Part model, mm, in its own coordinate system. A direction names the side the tool comes from. Give positions to 0.01 mm unless a question says otherwise; leave off trailing zeros. Order: outer loops, then holes, each group sorted by start corner. A loop starts at its lowest first (then second) coordinate and runs counter-clockwise, first axis right, second up. Notation, with made-up numbers: M -19,-21.75 L 29,-21.75 A21 cw 29,-9.75 Z; hole C 64,53.25 d10. An arc over 180 degrees is marked long. Answer as a JSON object with one key per item and string values.
from build123d import *

# Parameters (mm, degrees)
PAD001_DEPTH         = 40
SKETCH018_R          = 1.5
HOLE_DEPTH           = 4.5
HOLE_TIPS_R          = 1.5
SKETCH002_R          = 1.5
HOLE001_DEPTH        = 4.5
HOLE001_TIPS_R       = 1.5
SKETCH003_R          = 11
PAD002_DEPTH         = 2
PAD003_DEPTH         = 22
SKETCH005_R          = 2.5
PAD004_DEPTH         = 3
SKETCH006_W          = 16
SKETCH006_H          = 4
PAD005_DEPTH         = 2.5
PAD006_DEPTH         = 5
SKETCH008_W          = 0.5
SKETCH008_H          = 0.5
PAD007_DEPTH         = 4
BODY_PLACEMENT_ANGLE = 90


with BuildPart() as part:
    # Sketch017 → Pad001 (new body)
    with BuildSketch(Plane.XY):
        Polygon((-17.614466, 21.15), (17.614466, 21.15), (21.15, 17.614466), (21.15, -17.614466), (17.614466, -21.15), (-17.614466, -21.15), (-21.15, -17.614466), (-21.15, 17.614466), align=None)
    extrude(amount=PAD001_DEPTH)

    # Sketch018 (on Face10 of Pad001) → Hole (cut)
    with BuildSketch(Plane.XY.offset(40)):
        with Locations((15.5, 15.5)):
            Circle(SKETCH018_R)
        with Locations((-15.5, 15.5)):
            Circle(SKETCH018_R)
        with Locations((-15.5, -15.5)):
            Circle(SKETCH018_R)
        with Locations((15.5, -15.5)):
            Circle(SKETCH018_R)
    extrude(amount=-HOLE_DEPTH, mode=Mode.SUBTRACT)

    # Hole tips → Hole tip 1 section 0
    with BuildSketch(Plane.XY.offset(35.5), mode=Mode.PRIVATE) as hole_tip_1_s0:
        with Locations((15.5, 15.5)):
            Circle(HOLE_TIPS_R)
    loft([hole_tip_1_s0.sketch, Vertex(15.5, 15.5, 34.598709)], mode=Mode.SUBTRACT)

    # Hole tips → Hole tip 2 section 0
    with BuildSketch(Plane.XY.offset(35.5), mode=Mode.PRIVATE) as hole_tip_2_s0:
        with Locations((-15.5, 15.5)):
            Circle(HOLE_TIPS_R)
    loft([hole_tip_2_s0.sketch, Vertex(-15.5, 15.5, 34.598709)], mode=Mode.SUBTRACT)

    # Hole tips → Hole tip 3 section 0
    with BuildSketch(Plane.XY.offset(35.5), mode=Mode.PRIVATE) as hole_tip_3_s0:
        with Locations((-15.5, -15.5)):
            Circle(HOLE_TIPS_R)
    loft([hole_tip_3_s0.sketch, Vertex(-15.5, -15.5, 34.598709)], mode=Mode.SUBTRACT)

    # Hole tips → Hole tip 4 section 0
    with BuildSketch(Plane.XY.offset(35.5), mode=Mode.PRIVATE) as hole_tip_4_s0:
        with Locations((15.5, -15.5)):
            Circle(HOLE_TIPS_R)
    loft([hole_tip_4_s0.sketch, Vertex(15.5, -15.5, 34.598709)], mode=Mode.SUBTRACT)

    # Sketch002 → Hole001 (cut)
    with BuildSketch(Plane.XY):
        with Locations((-15.5, 15.5)):
            Circle(SKETCH002_R)
        with Locations((-15.5, -15.5)):
            Circle(SKETCH002_R)
        with Locations((15.5, -15.5)):
            Circle(SKETCH002_R)
        with Locations((15.5, 15.5)):
            Circle(SKETCH002_R)
    extrude(amount=HOLE001_DEPTH, mode=Mode.SUBTRACT)

    # Hole001 tips → Hole001 tip 1 section 0
    with BuildSketch(Plane.XY.offset(4.5), mode=Mode.PRIVATE) as hole001_tip_1_s0:
        with Locations((-15.5, 15.5)):
            Circle(HOLE001_TIPS_R)
    loft([hole001_tip_1_s0.sketch, Vertex(-15.5, 15.5, 5.401291)], mode=Mode.SUBTRACT)

    # Hole001 tips → Hole001 tip 2 section 0
    with BuildSketch(Plane.XY.offset(4.5), mode=Mode.PRIVATE) as hole001_tip_2_s0:
        with Locations((-15.5, -15.5)):
            Circle(HOLE001_TIPS_R)
    loft([hole001_tip_2_s0.sketch, Vertex(-15.5, -15.5, 5.401291)], mode=Mode.SUBTRACT)

    # Hole001 tips → Hole001 tip 3 section 0
    with BuildSketch(Plane.XY.offset(4.5), mode=Mode.PRIVATE) as hole001_tip_3_s0:
        with Locations((15.5, -15.5)):
            Circle(HOLE001_TIPS_R)
    loft([hole001_tip_3_s0.sketch, Vertex(15.5, -15.5, 5.401291)], mode=Mode.SUBTRACT)

    # Hole001 tips → Hole001 tip 4 section 0
    with BuildSketch(Plane.XY.offset(4.5), mode=Mode.PRIVATE) as hole001_tip_4_s0:
        with Locations((15.5, 15.5)):
            Circle(HOLE001_TIPS_R)
    loft([hole001_tip_4_s0.sketch, Vertex(15.5, 15.5, 5.401291)], mode=Mode.SUBTRACT)

    # Sketch003 (on Face5 of Hole001) → Pad002 (join)
    with BuildSketch(Plane.XY.offset(40)):
        Circle(SKETCH003_R)
    extrude(amount=PAD002_DEPTH)

    # Sketch004 (on Face27 of Pad002) → Pad003 (join)
    with BuildSketch(Plane.XY.offset(42)):
        with BuildLine():
            ThreePointArc((-1.5, 2), (0, -2.5), (1.5, 2))
            Line((-1.5, 2), (1.5, 2))
        make_face()
    extrude(amount=PAD003_DEPTH)

    # Sketch005 (on Face27 of Pad002) → Pad004 (join)
    with BuildSketch(Plane.XY.offset(42)):
        Circle(SKETCH005_R)
    extrude(amount=PAD004_DEPTH)

    # Sketch006 (on Face4 of Pad004) → Pad005 (join)
    with BuildSketch(Plane(origin=(0, 0, 0), x_dir=(1, 0, 0), z_dir=(0, 0, -1))):
        with Locations((0, 23.15)):
            Rectangle(SKETCH006_W, SKETCH006_H)
    extrude(amount=-PAD005_DEPTH)

    # Sketch007 (on Face10 of Pad005) → Pad006 (join)
    with BuildSketch(Plane.XZ.offset(21.15)):
        Polygon((-4.2, 9), (-8, 9), (-8, 2.5), (8, 2.5), (8, 9), (4.2, 9), (4.2, 8.4), (7.4, 8.4), (7.4, 3.1), (-7.4, 3.1), (-7.4, 8.4), (-4.2, 8.4), align=None)
    extrude(amount=PAD006_DEPTH)

    # Sketch008 (on Face10 of Pad006) → Pad007 (join)
    with BuildSketch(Plane.XZ.offset(21.15)):
        with Locations((-5.25, 6.35)):
            Rectangle(SKETCH008_W, SKETCH008_H)
        with Locations((-3.15, 6.35)):
            Rectangle(SKETCH008_W, SKETCH008_H)
        with Locations((-1.05, 6.35)):
            Rectangle(SKETCH008_W, SKETCH008_H)
        with Locations((1.05, 6.35)):
            Rectangle(SKETCH008_W, SKETCH008_H)
        with Locations((3.15, 6.35)):
            Rectangle(SKETCH008_W, SKETCH008_H)
        with Locations((5.25, 6.35)):
            Rectangle(SKETCH008_W, SKETCH008_H)
    extrude(amount=PAD007_DEPTH)


with BuildPart() as part_1:
    # Body placement: moved
    add(part.part.rotate(Axis((0, 0, 0), (0, -1, 0)), BODY_PLACEMENT_ANGLE))


solid = part_1.part
1. Cut at A-A on z = 0. Give the cut face in (x, y), plus the area to 3 significant figures.
Worked answers:
{"outline": "M -64,-2.5 L -42,-2.5 L -42,-11 L -40,-11 L -40,-21.15 L -3.1,-21.15 L -3.1,-26.15 L -2.5,-26.15 L -2.5,-25.15 L 0,-25.15 L 0,21.15 L -40,21.15 L -40,11 L -42,11 L -42,2.5 L -45,2.5 L -45,2 L -64,2 Z", "area": "1,850 mm^2"}
2. Probe line 1 along Y through (x, z) = (-39.05, -15.5); line 2 along Z through (x, y) = (-2, 15). List the from-to ranges inside material, lowest first.
Worked answers:
{"line 1": "y = -21.15 to -17, -14 to 14, 17 to 21.15", "line 2": "z = -21.15 to -16.91, -14.09 to 14.09, 16.91 to 21.15"}
3. Two-plate mould, pull along Z, no slides. Class faces 5 (the flat face through (-9, -24, -6)), 6 (the conical face through (-34.743, 15.572, 15.728)), 7 (the flat face through (-20, 0, -21.15)): +Z half, -Z half, draft (parallel to the pull), parting line (faces both ways), or undercut.
Worked answers:
{"face 5": "draft", "face 6": "undercut", "face 7": "-Z half"}
4. Cut at D-D on y = 9.5. Give the cut face in (x, z).
Worked answers:
{"outline": "M -42,-5.55 L -40,-5.55 L -40,-21.15 L 0,-21.15 L 0,21.15 L -40,21.15 L -40,5.55 L -42,5.55 Z"}
5. Cut at C-C on y = 0. Give the cut face in (x, z).
Worked answers:
{"outline": "M -64,-2.5 L -42,-2.5 L -42,-11 L -40,-11 L -40,-21.15 L 0,-21.15 L 0,21.15 L -40,21.15 L -40,11 L -42,11 L -42,2.5 L -64,2.5 Z"}
6. Pin check, flat tips, straight feed: P1, Ø5, axis at y = 12, z = -4, coming from the -X side; P2, Ø3.5, axis at y = -15.5, z = 15.5, coming from the -X side; P3, Ø6, axis at x = -18.5, z = -1.5, coming from the -Y side; P4, Ø6, axis at x = -46, y = 12.5, coming from the -Z side. Stop position of each tip, or through.
Worked answers:
{"P1": "stops at x = -42", "P2": "stops at x = -40", "P3": "stops at y = -21.15", "P4": "passes through"}
7. Which spindle directions (+Z, -Z, +X, -X, +Y, -Y) get a long thin tool onto all of the face, cutting with end or side? Do faces 1 (the flat face through (-6, -24, -7.4)), 2 (the flat face through (-4, -24, 8)), 3 (the flat face through (-40, 10, -9)), 4 (the flat face through (-1, -25.15, 0)). Say none if no direction does.
Worked answers:
{"face 1": "-Y", "face 2": "+Z, +X, -X, -Y", "face 3": "-X", "face 4": "+Z, -Z, +X, -Y"}
8. Cut at B-B on x = -21.5. Give the cut face in (y, z), plus the area to 3 significant figures.
Worked answers:
{"outline": "M -21.15,-17.61 L -17.61,-21.15 L 17.61,-21.15 L 21.15,-17.61 L 21.15,17.61 L 17.61,21.15 L -17.61,21.15 L -21.15,17.61 Z", "area": "1,760 mm^2"}
